For this review, take the finished solid that the model builds, in its own axes (mm). Give positions to 0.01 mm unless a question says otherwise; leave off trailing zeros. Write each loop counter-clockwise with the first axis right and the second up, starting at its lowest first coordinate (ties: lowest second). Pieces come first, ordered by that corner, then holes. Notation, with made-up numbers: M -25,49.5 L 16,49.5 A18 ccw 16,73.5 Z; hole C 43.5,4 d4. An arc over 180 degrees is marked long. Answer as a JSON object with one key per item and string values. Group by question number.
Autodesk Inventor part; units mm, degrees
ref_plane "YZ Plane" through (0, 0, 0) normal (1, 0, 0) x (0, 1, 0)
ref_plane "XZ Plane" through (0, 0, 0) normal (0, 1, 0) x (-1, 0, 0)
ref_plane "XY Plane" through (0, 0, 0) normal (0, 0, 1) x (1, 0, 0)
sketch "Skizze1" plane through (0, 0, 0) normal (0, 0, 1) x (1, 0, 0)
  circle A0 centre (0, 0) radius 60
  circle A1 centre (0, 0) radius 43.5 construction
  circle A2 centre (0, 43.5) radius 1.7
  circle A3 centre (37.6721, -21.75) radius 1.7
  circle A4 centre (-37.6721, -21.75) radius 1.7
  line L0 (0, 0) -> (37.6721, -21.75) construction
  line L1 (0, 0) -> (-37.6721, -21.75) construction
  line L2 (0, 84) -> (0, -84) construction
  line L3 (-84, 0) -> (84, 0) construction
  dimension "d0" = 120
  dimension "d1" = 87
  dimension "d2" = 3.4
  dimension "d3" = 120
extrude "Extrusion1" add sketch "Skizze1" along normal blind 3
fillet "Rundung1" radius 1 2 edges at (-60, 0, 3) (-60, 0, 0)
properties part number "Base-Plate"
Item 1: Draft analysis for pull direction Y (two halves, no side actions). For faces 1 (the flat face through (-1, 1, 3)), 2 (the cylindrical face through (-39.37, -21.82, 1.48)), 3 (the cylindrical face through (-59.94, -2.64, 1.49)), state which applies: released by +Y, released by -Y, zero draft, split by the parting line, or undercut.
Item 2: Consider section A-A (y = -21.75). State how many separate pieces and enclosed holes the cut face has, plus the area to 3 significant figures.
Item 3: Consider section B-B (z = 0.5). Give the boundary of the cut face in (x, y).
Item 4: Insertion check: P1, Ø1, axis at y = -1, z = 1, coming from the +X side; P2, Ø3, axis at x = 0, y = 43.5, coming from the -Z side; P3, Ø1.5, axis at x = -43, z = 0.5, coming from the +Y side. Each pin has a flat end and moves straight along its axis. Give the tip position at first contact, or say it passes through.
Item 5: To check wall thickness, follow probe 1 along X at (y, z) = (-21, 2.3); probe 2 along Y at (x, z) = (29.5, 1.8); probe 3 along X at (y, z) = (-32.5, 2.5). State the ranges of each line that lie inside material, in increasing order.
Result set:
{
 "1": {"face 1": "zero draft", "face 2": "undercut", "face 3": "split by the parting line"},
 "2": {"separate pieces": "3", "enclosed holes": "0", "area": "314 mm^2"},
 "3": {"outline": "C 0,0 d119.73; hole C -37.67,-21.75 d3.4; hole C 0,43.5 d3.4; hole C 37.67,-21.75 d3.4"},
 "4": {"P1": "stops at x = 60", "P2": "passes through", "P3": "stops at y = 42.51"},
 "5": {"probe 1": "x = -56.16 to -39.2, -36.15 to 36.15, 39.2 to 56.16", "probe 2": "y = -52.25 to 52.25", "probe 3": "x = -50.28 to 50.28"}
}
